Source: CAD feature listing. Evaluate the final solid. Frame: model axes, mm. A direction names the side the tool comes from. Coordinates: 2 decimals unless noted, no trailing zeros. Order: outer loops, then holes, each group sorted by start corner. A loop starts at its lowest first (then second) coordinate and runs counter-clockwise, first axis right, second up.
```python
from build123d import *

# Parameters (mm, degrees)
F0_R     = 2.2479
F0_R_2   = 11
F1_DEPTH = 3.175
F2_R     = 11
F3_DEPTH = 3.8250114
F4_R     = 11
F4_R_2   = 9.4125034
F5_DEPTH = 1.5875
F7_DEPTH = 8.5875114


with BuildPart() as f1:
    # F0 (on Top) → F1 (new body)
    with BuildSketch(Plane.XY):
        with BuildLine():
            Line((3.96875, -18.14374959), (3.96875, -13.6080724871))
            ThreePointArc((3.96875, -13.6080724871), (14.17499959, 0), (3.96875, 13.6080724871))
            Line((3.96875, 13.6080724871), (3.96875, 18.14374959))
            ThreePointArc((3.96875, 18.14374959), (0, 22.11249959), (-3.96875, 18.14374959))
            Line((-3.96875, 18.14374959), (-3.96875, 13.6080724871))
            ThreePointArc((-3.96875, 13.6080724871), (-14.17499959, 0), (-3.96875, -13.6080724871))
            Line((-3.96875, -13.6080724871), (-3.96875, -18.14374959))
            ThreePointArc((-3.96875, -18.14374959), (0, -22.11249959), (3.96875, -18.14374959))
        make_face()
        with Locations((0, -18.14374959)):
            Circle(F0_R, mode=Mode.SUBTRACT)
        Circle(F0_R_2, mode=Mode.SUBTRACT)
        with Locations((0, 18.14374959)):
            Circle(F0_R, mode=Mode.SUBTRACT)
    extrude(amount=F1_DEPTH)

    # F2 (on face) → F3 (join)
    with BuildSketch(Plane.XY.offset(3.175)):
        with BuildLine():
            ThreePointArc((2.38125, 14.96874959), (0, 14.17499959), (-2.38125, 14.96874959))
            Line((-2.38125, 14.96874959), (-3.96875, 14.96874959))
            Line((-3.96875, 14.96874959), (-3.96875, 13.6080724871))
            ThreePointArc((-3.96875, 13.6080724871), (-14.17499959, 0), (-3.96875, -13.6080724871))
            Line((-3.96875, -13.6080724871), (-3.96875, -14.96874959))
            Line((-3.96875, -14.96874959), (-2.38125, -14.96874959))
            ThreePointArc((-2.38125, -14.96874959), (0, -14.17499959), (2.38125, -14.96874959))
            Line((2.38125, -14.96874959), (3.96875, -14.96874959))
            Line((3.96875, -14.96874959), (3.96875, -13.6080724871))
            ThreePointArc((3.96875, -13.6080724871), (14.17499959, 0), (3.96875, 13.6080724871))
            Line((3.96875, 13.6080724871), (3.96875, 14.96874959))
            Line((3.96875, 14.96874959), (2.38125, 14.96874959))
        make_face()
        Circle(F2_R, mode=Mode.SUBTRACT)
    extrude(amount=F3_DEPTH)

    # F4 (on face) → F5 (join)
    with BuildSketch(Plane.XY.offset(7.0000114)):
        with BuildLine():
            ThreePointArc((3.96875, -13.6080724871), (14.17499959, 0), (3.96875, 13.6080724871))
            Line((3.96875, 13.6080724871), (3.96875, 14.96874959))
            Line((3.96875, 14.96874959), (2.38125, 14.96874959))
            ThreePointArc((2.38125, 14.96874959), (0, 14.17499959), (-2.38125, 14.96874959))
            Line((-2.38125, 14.96874959), (-3.96875, 14.96874959))
            Line((-3.96875, 14.96874959), (-3.96875, 13.6080724871))
            ThreePointArc((-3.96875, 13.6080724871), (-14.17499959, 0), (-3.96875, -13.6080724871))
            Line((-3.96875, -13.6080724871), (-3.96875, -14.96874959))
            Line((-3.96875, -14.96874959), (-2.38125, -14.96874959))
            ThreePointArc((-2.38125, -14.96874959), (0, -14.17499959), (2.38125, -14.96874959))
            Line((2.38125, -14.96874959), (3.96875, -14.96874959))
            Line((3.96875, -14.96874959), (3.96875, -13.6080724871))
        make_face()
        Circle(F4_R, mode=Mode.SUBTRACT)
        Circle(F4_R)
        Circle(F4_R_2, mode=Mode.SUBTRACT)
    extrude(amount=F5_DEPTH)

    # F6 (on face) → F7 (join, through all)
    with BuildSketch(Plane.XY.offset(8.5875114)):
        with BuildLine():
            ThreePointArc((-3.96875, 14.96874959), (-4.2997839234, 13.8956272964), (-5.1778315745, 13.1954792851))
            ThreePointArc((-5.1778315745, 13.1954792851), (-4.57794134, 13.4154040738), (-3.96875, 13.6080724871))
            Line((-3.96875, 13.6080724871), (-3.96875, 14.96874959))
        make_face()
        with BuildLine():
            ThreePointArc((5.1778315745, 13.1954792851), (4.2997839234, 13.8956272964), (3.96875, 14.96874959))
            Line((3.96875, 14.96874959), (3.96875, 13.6080724871))
            ThreePointArc((3.96875, 13.6080724871), (4.57794134, 13.4154040738), (5.1778315745, 13.1954792851))
        make_face()
        with BuildLine():
            ThreePointArc((-5.1778315745, -13.1954792851), (-4.2997839234, -13.8956272964), (-3.96875, -14.96874959))
            Line((-3.96875, -14.96874959), (-3.96875, -13.6080724871))
            ThreePointArc((-3.96875, -13.6080724871), (-4.57794134, -13.4154040738), (-5.1778315745, -13.1954792851))
        make_face()
        with BuildLine():
            ThreePointArc((3.96875, -14.96874959), (4.2997839234, -13.8956272964), (5.1778315745, -13.1954792851))
            ThreePointArc((5.1778315745, -13.1954792851), (4.57794134, -13.4154040738), (3.96875, -13.6080724871))
            Line((3.96875, -13.6080724871), (3.96875, -14.96874959))
        make_face()
    extrude(amount=-F7_DEPTH)


solid = f1.part
```
1. Section query C-C on y = 0. Return loops of the section in (x, z) (1 decimal), plus the area to 3 significant figures.
Findings:
outline: (-14.2, 0) - (-11, 0) - (-11, 7) - (-9.4, 7) - (-9.4, 8.6) - (-14.2, 8.6) - close; (9.4, 7) - (11, 7) - (11, 0) - (14.2, 0) - (14.2, 8.6) - (9.4, 8.6) - close
area: 59.6 mm2
2. Section query D-D on x = -3.25. Return loops of the section in (y, z) (3 decimals), plus the area to 3 significant figures.
Findings:
outline: (-20.422, 0) - (-10.509, 0) - (-10.509, 7) - (-8.834, 7) - (-8.834, 8.588) - (-14.969, 8.588) - (-14.969, 3.175) - (-20.422, 3.175) - close; (8.834, 7) - (10.509, 7) - (10.509, 0) - (20.422, 0) - (20.422, 3.175) - (14.969, 3.175) - (14.969, 8.588) - (8.834, 8.588) - close
area: 117 mm2
3. Access query for faces 1 (the face through (-0.036, -14.175, 5.843)), 2 (the face through (-3.969, 17, 2)), 3 (the face through (3, -14.969, 6)). Directions: +Z, -Z, +X, -X, +Y, -Y. A direction counts if a zero-diameter tool reaches every point of the face in a straight line with its end or side. Return the directions, or none.
Findings:
face 1: +Z, -Y
face 2: +Z, -Z, -X, +Y
face 3: +Z, +X, -X, -Y
4. Draft query along X for faces 4 (the face through (14.173, -0.238, 4.234)), 5 (the face through (0.036, 14.175, 5.843)), 6 (the face through (-0.09, -22.11, 1.57)). Return one class per face: released by +X, released by -X, zero draft, split by the parting line, or undercut.
Findings:
face 4: released by +X
face 5: undercut
face 6: split by the parting line
5. Pin query (flat end, axial travel): P1, Ø3, axis at x = 10.5, z = 1.5, coming from the -Y side; P2, Ø2.5, axis at x = 0, y = 18.14, coming from the +Z side; P3, Ø4, axis at x = -0.5, y = 19, coming from the +Z side (3 decimals); P4, Ø3.5, axis at y = -17, z = 2, coming from the +X side. Return the tip coordinate at first contact, or that it passes through.
Findings:
P1: stops at y = -10.95
P2: passes through
P3: stops at z = 3.175
P4: stops at x = 3.97
6. Ray query, line 1 (Y direction, x = 0, z = 2.35); line 2 (Y direction, x = -1, z = 1.25); line 3 (Y direction, x = 0, z = 4.25) (3 decimals). Return the intervals inside material, ascending.
Findings:
line 1: y = -22.11 to -20.39, -15.9 to -11, 11 to 15.9, 20.39 to 22.11
line 2: y = -21.98 to -20.16, -16.13 to -10.95, 10.95 to 16.13, 20.16 to 21.98
line 3: y = -14.175 to -11, 11 to 14.175
7. Section query A-A on x = 0. Return loops of the section in (y, z) (1 decimal), plus the area to 3 significant figures.
Findings:
outline: (-22.1, 0) - (-20.4, 0) - (-20.4, 3.2) - (-22.1, 3.2) - close; (-15.9, 0) - (-11, 0) - (-11, 7) - (-9.4, 7) - (-9.4, 8.6) - (-14.2, 8.6) - (-14.2, 3.2) - (-15.9, 3.2) - close; (9.4, 7) - (11, 7) - (11, 0) - (15.9, 0) - (15.9, 3.2) - (14.2, 3.2) - (14.2, 8.6) - (9.4, 8.6) - close; (20.4, 0) - (22.1, 0) - (22.1, 3.2) - (20.4, 3.2) - close
area: 81.4 mm2
